Geometry: see drawing. Coordinates: mm, zero at the bounding-box minimum. A direction names the side the tool comes from. Round coordinates to 2 decimals unless told otherwise and drop trailing zeros. Write each loop counter-clockwise with the first axis right and the second up, starting at its lowest first coordinate (ties: lowest second). Pieces come first, ordered by that corner, then holes.
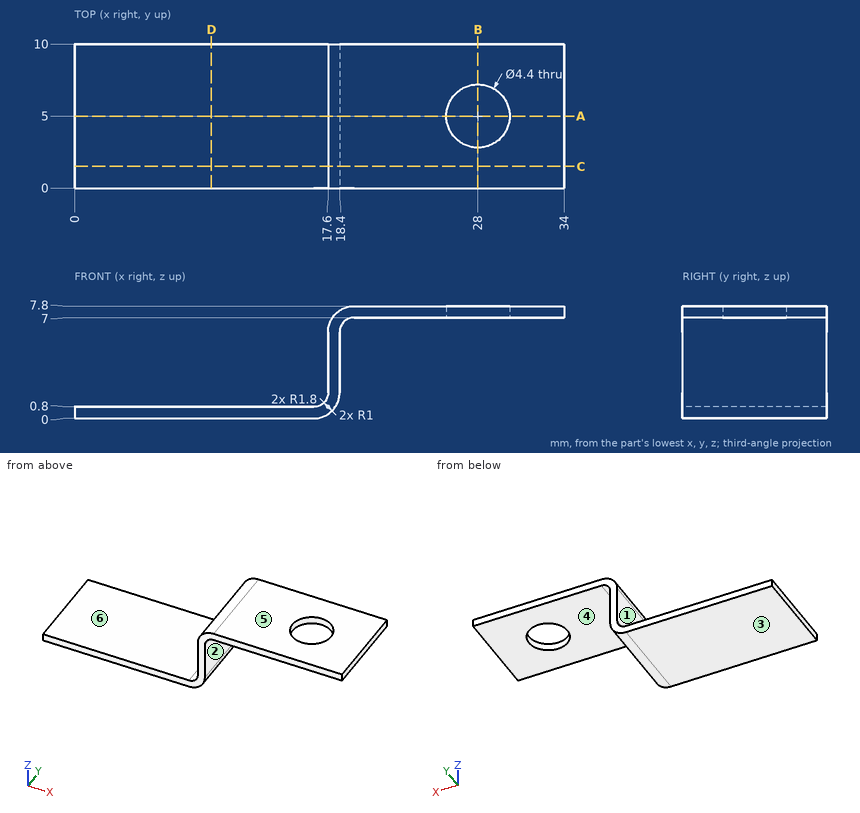
1) Pull-direction query (X, two-part tool) for the marked faces 1, 2 and 3; classes: released by +X, released by -X, zero draft, split by the parting line, or undercut.
Taken from the geometry:
face 1: released by -X
face 2: released by +X
face 3: zero draft
2) Contact query for flat-ended pins moving along their axis: P1, Ø1, axis at y = 5, z = 4.5, coming from the +X side; P2, Ø1.3, axis at y = 6, z = 4.5, coming from the -X side; P3, Ø5, axis at x = 24, y = 5, coming from the -Z side. Output: stop coordinate, or through.
Taken from the geometry:
P1: stops at x = 18.4
P2: stops at x = 17.6
P3: stops at z = 7
3) Section query C-C on y = 1.5. Return the cut outline in (x, z), then the cut area to 3 significant figures.
Taken from the geometry:
outline: (0, 0) - (16.6, 0) arc R1.8 ccw to (18.4, 1.8) - (18.4, 6) arc R1 cw to (19.4, 7) - (34, 7) - (34, 7.8) - (19.4, 7.8) arc R1.8 ccw to (17.6, 6) - (17.6, 1.8) arc R1 cw to (16.6, 0.8) - (0, 0.8) - close
area: 31.8 mm2
4) Section query D-D on x = 9.5. Return the cut outline in (y, z), then the cut area to 3 significant figures.
Taken from the geometry:
outline: (0, 0) - (10, 0) - (10, 0.8) - (0, 0.8) - close
area: 8.00 mm2
5) Section query A-A on y = 5. Return the cut outline in (x, z), then the cut area to 3 significant figures.
Taken from the geometry:
outline: (0, 0) - (16.6, 0) arc R1.8 ccw to (18.4, 1.8) - (18.4, 6) arc R1 cw to (19.4, 7) - (25.8, 7) - (25.8, 7.8) - (19.4, 7.8) arc R1.8 ccw to (17.6, 6) - (17.6, 1.8) arc R1 cw to (16.6, 0.8) - (0, 0.8) - close; (30.2, 7) - (34, 7) - (34, 7.8) - (30.2, 7.8) - close
area: 28.3 mm2
6) Section query B-B on x = 28. Return the cut outline in (y, z), then the cut area to 3 significant figures.
Taken from the geometry:
outline: (0, 7) - (2.8, 7) - (2.8, 7.8) - (0, 7.8) - close; (7.2, 7) - (10, 7) - (10, 7.8) - (7.2, 7.8) - close
area: 4.48 mm2
7) Reachability of the marked faces 4, 5 and 6 from +Z, -Z, +X, -X, +Y, -Y: full face, straight path, thin tool, end or side. Return the list, or none.
Taken from the geometry:
face 4: -Z, +X, +Y, -Y
face 5: +Z, +X, -X, +Y, -Y
face 6: +Z, -X, +Y, -Y
8) Material intervals for line 1 (Y direction, x = 28, z = 7.5); line 2 (Z direction, x = 25, y = 7.5); line 3 (Z direction, x = 9, y = 5), sorted ascending.
Taken from the geometry:
line 1: y = 0 to 2.8, 7.2 to 10
line 2: z = 7 to 7.8
line 3: z = 0 to 0.8
